Can you work these out from the model? Positions are in its coordinate system, mm. A direction names the side the tool comes from. Give positions to 0.01 mm unless a question says otherwise; leave off trailing zeros. Write each loop counter-clockwise with the first axis right and the second up, starting at its lowest first coordinate (ties: lowest second). Pieces come first, ordered by that corner, then holes. Notation, with made-up numbers: (-2, -15.75) -> (57, -15.75) arc R16 ccw to (57, 0.25) -> close; hole circle Ø2 at (-13.5, 70.25). An arc over 180 degrees is marked (long way). Answer as CSV lines item,"result". Start each with the question number.
1. If we section it at B-B on y = -2.25: Write out the boundary of the cut face in (x, z) (3 decimals).
2. If we section it at A-A on y = 3.5: Write out the boundary of the cut face in (x, z) (3 decimals), plus the area to 3 significant figures.
3. On a 3-axis mill with a long thin cutter (end or side, diameter ignored), from which of +Z, -Z, +X, -X, +Y, -Y can I reach the whole of each face in a straight line? I mean faces 4 (the face through (11.99, 5.498, 1.565)), 5 (the face through (8.296, 4.103, 1.565)). Say none if no direction works.
4. If we section it at C-C on x = 18.25: Write out the boundary of the cut face in (y, z) (3 decimals).
5. I need wall thicknesses on line 1 (X direction, y = 2.5, z = 0.6); line 2 (X direction, y = 3, z = 1.9); line 3 (Y direction, x = 8.5, z = 2.8). Which ranges of each line are inside material? Lowest first, please. Write a range as [from, to].
6. If we section it at D-D on z = 1.65: Count the separate pieces of the cut face and the enclosed holes in it, plus the area to 3 significant figures.
7. If we mould it in two halves opening along X, with no side actions, what happens to faces 1 (the face through (11.14, -5.95, 1.61)), 2 (the face through (7.521, -5.126, 1.61)), 3 (the face through (16.77, 3.15, 1.57))? For each: pulls with the +X half, pulls with the -X half, needs draft (parallel to the pull), parting line crosses it, or undercut.
Autodesk Inventor part; units mm, degrees
ref_plane "YZ Plane" through (0, 0, 0) normal (1, 0, 0) x (0, 1, 0)
ref_plane "XZ Plane" through (0, 0, 0) normal (0, 1, 0) x (-1, 0, 0)
ref_plane "XY Plane" through (0, 0, 0) normal (0, 0, 1) x (1, 0, 0)
sketch "Sketch1" plane through (0, 0, 0) normal (0, 0, 1) x (1, 0, 0)
  line L0 (6.8234, 3.035) -> (6.5538, -6.1146)
  line L1 (6.5538, -6.1146) -> (11.2152, -6.1146)
  line L2 (11.2152, -6.1146) -> (20.3343, 0.9713)
  circle A0 centre (18.3549, 3.2173) radius 2.9937
  circle A1 centre (18.3549, 3.2173) radius 1.5875
  line L3 (18.9975, 6.1413) -> (13.9136, 5.1722)
  circle A2 centre (9.5555, 3.1371) radius 2.734
  circle A3 centre (9.5555, 3.1371) radius 1.5875
  line L4 (13.9136, 5.1722) -> (10.0118, 5.8327)
  point P0 (0, 0)
  dimension "d0" = 3.175
  dimension "d1" = 3.175
extrude "Extrusion1" add sketch "Sketch1" along normal blind 3.175 contours A2 L4 L3 A0 L2 L1 L0 | A2 | A0 L3 L2
sketch "Sketch2" plane through (0, 0, 3.175) normal (0, 0, 1) x (1, 0, 0)
  circle A0 centre (9.525, -3.175) radius 1.5875
  point P0 (0, 0)
extrude "Extrusion2" cut sketch "Sketch2" against normal blind 3.175
fillet "Fillet1" radius 3.175 2 edges at (6.5538, -6.1146, 1.5875) (11.2152, -6.1146, 1.5875)
properties part number "UpperLever"
Computed values:
1,outline,"(6.668, 0) -> (8.235, 0) -> (8.235, 3.175) -> (6.668, 3.175) -> close; (10.815, 0) -> (16.189, 0) -> (16.189, 3.175) -> (10.815, 3.175) -> close"
2,outline,"(6.846, 0) -> (8.01, 0) -> (8.01, 3.175) -> (6.846, 3.175) -> close; (11.101, 0) -> (16.793, 0) -> (16.793, 3.175) -> (11.101, 3.175) -> close; (19.917, 0) -> (21.335, 0) -> (21.335, 3.175) -> (19.917, 3.175) -> close"
2,area,"26.3 mm2"
3,face 4,"+Z, -Z, +Y"
3,face 5,"+Z, -Z"
4,outline,"(-0.648, 0) -> (1.633, 0) -> (1.633, 3.175) -> (-0.648, 3.175) -> close; (4.801, 0) -> (5.999, 0) -> (5.999, 3.175) -> (4.801, 3.175) -> close"
5,line 1,"x = [6.81, 8.1], [11.01, 16.94], [19.77, 21.26]"
5,line 2,"x = [6.82, 7.97], [11.14, 16.78], [19.93, 21.34]"
5,line 3,"y = [-5.83, -4.39], [-1.96, 1.95], [4.32, 5.66]"
6,separate pieces,"1"
6,enclosed holes,"3"
6,area,"104 mm2"
7,face 1,"pulls with the +X half"
7,face 2,"pulls with the -X half"
7,face 3,"undercut"
